```python
from build123d import *

# Parameters (mm, degrees)
SKETCH1_R           = 12.7
BOSS_EXTRUDE1_DEPTH = 152.4
SKETCH5_R           = 12.7
BOSS_EXTRUDE3_DEPTH = 106
SKETCH6_W           = 7.5
SKETCH6_H           = 20.5
BOSS_EXTRUDE5_DEPTH = 30
SKETCH7_R           = 3.675
CUT_EXTRUDE1_DEPTH  = 152.4


with BuildPart() as part:
    # Sketch1 → Boss-Extrude1 (new body)
    with BuildSketch(Plane(origin=(0, 0, 0), x_dir=(0, 0, -1), z_dir=(1, 0, 0))):
        with Locations(Location((0, 0, 0), (0, 0, 180))):
            Circle(SKETCH1_R)
    extrude(amount=BOSS_EXTRUDE1_DEPTH)

    # Sketch5 → Boss-Extrude3 (add)
    with BuildSketch(Plane(origin=(31.75, 31.75, 0), x_dir=(0.7071067811865464, -0.7071067811865488, 0), z_dir=(0.7071067811865488, 0.7071067811865464, 0))):
        with Locations(Location((44.901280605, 0, 0), (0, 0, 90))):
            Circle(SKETCH5_R)
    extrude(amount=BOSS_EXTRUDE3_DEPTH)

    # Sketch6 → Boss-Extrude5 (add)
    with BuildSketch(Plane(origin=(106.703318806, 106.703318806, 0), x_dir=(0, 0, -1), z_dir=(0.7071067811865487, 0.7071067811865465, 0))):
        with Locations((-3.75, -44.901280605)):
            Rectangle(SKETCH6_W, SKETCH6_H)
    extrude(amount=BOSS_EXTRUDE5_DEPTH)

    # Sketch7 → Cut-Extrude1 (cut)
    with BuildSketch(Plane.ZY):
        Circle(SKETCH7_R)
    extrude(amount=-CUT_EXTRUDE1_DEPTH, mode=Mode.SUBTRACT)


solid = part.part
```
Can you work these out from the model? Positions are in its coordinate system, mm. A direction names the side the tool comes from. Round coordinates to 2 decimals unless told otherwise and drop trailing zeros. Loops run counter-clockwise (first coordinate to the right, second up) from the corner with the lowest first, then second, coordinate; pieces in that order, holes last. Notation, with made-up numbers: M -17,-40 L 37,-40 A12 ccw 37,-23 Z; hole C 63,37.5 d5. An arc over 180 degrees is marked long. Answer as a JSON object with one key per item and string values. Group by question number.
Q1. Imagine slicing it at B-B, the plane z = -6. Please give me the cut outline in (x, y), then the cut area to 3 significant figures.
Q2. Imagine slicing it at C-C, the plane y = 93.5. Please give me the cut outline in (x, z), then the cut area to 3 significant figures.
Q3. We'd pull the mould along Y, two halves only. Please class faces 4 (the flat face through (156.159, 78.164, 3.802)), 5 (the flat face through (149, 85, 7.5)), 6 (the cylindrical face through (75.133, -12.592, -1.653)), 7 (the flat face through (138.352, 75.055, 9.559)): +Y half, -Y half, draft (parallel to the pull), parting line (faces both ways), or undercut.
Q4. Will these pins go through, and if not, where does the flat tip stop? pin 1 (6.5 mm diameter, centred on y = 0, z = 0, fed in from -X); pin 2 (4 mm diameter, centred on x = 95, y = 17, fed in from +Z); pin 3 (3 mm diameter, centred on x = 73, z = -8.5, fed in from +Y); pin 4 (10.5 mm diameter, centred on x = 149.5, y = 85.5, fed in from -Z).
Q5. Please list where these lines run through material, in increasing order: L1, parallel to Y at x = 113, z = 0 (3 decimals); L2, parallel to Y at x = 101, z = 0 (3 decimals); L3, parallel to X at y = 3.5, z = -8.
Q6. On a 3-axis mill with a long thin cutter (end or side, diameter ignored), from which of +Z, -Z, +X, -X, +Y, -Y can I reach the whole of each face in a straight line? I mean faces 1 (the flat face through (152.4, 3, 3)), 2 (the flat face through (149, 85, 0)), 3 (the flat face through (159.565, 96.268, 3.802)). Say none if no direction works.
Q7. Imagine slicing it at A-A, the plane x = 49. Please give me the cut outline in (y, z) (3 decimals).
Findings:
{
 "1": {"outline": "M 0,-11.19 L 152.4,-11.19 L 152.4,11.19 L 90.52,11.19 L 146.37,67.04 L 130.54,82.87 L 58.86,11.19 L 0,11.19 Z", "area": "5,430 mm2"},
 "2": {"outline": "M 142.5,0 L 162.33,0 L 162.33,7.5 L 142.5,7.5 Z", "area": "149 mm2"},
 "3": {"face 4": "undercut", "face 5": "draft", "face 6": "undercut", "face 7": "+Y half"},
 "4": {"pin 1": "passes through", "pin 2": "stops at z = 9.65", "pin 3": "stops at y = 25.12", "pin 4": "stops at z = 0"},
 "5": {"L1": "y = -12.7 to -3.675, 3.675 to 12.7, 31.539 to 67.461", "L2": "y = -12.7 to -3.675, 3.675 to 12.7, 19.539 to 55.461", "L3": "x = 0 to 152.4"},
 "6": {"face 1": "+Z, -Z, +X, -Y", "face 2": "-Z, +X, +Y", "face 3": "+Z, -Z, +X, +Y"},
 "7": {"outline": "C 0,0 d25.4; hole C 0,0 d7.35"}
}
